Input: part model. Units: mm. Frame: model coordinates. A direction names the side the tool comes from. Coordinates: 2 decimals unless noted, no trailing zeros. Loops run counter-clockwise (first coordinate to the right, second up) from the corner with the lowest first, then second, coordinate; pieces in that order, holes last.
```python
from build123d import *

# Parameters (mm, degrees)
F0_R     = 24
F1_DEPTH = 50
F2_R     = 65
F2_R_2   = 24
F3_DEPTH = 50
F4_R     = 15


with BuildPart() as f1:
    # F0 (on Top) → F1 (new body)
    with BuildSketch(Plane.XY):
        with BuildLine():
            ThreePointArc((67.890381, 85.131845), (54.235467, 112.621108), (24.229797, 106.157675))
            ThreePointArc((24.229797, 106.157675), (0, 125), (-24.229797, 106.157675))
            ThreePointArc((-24.229797, 106.157675), (-54.235467, 112.621108), (-67.890381, 85.131845))
            ThreePointArc((-67.890381, 85.131845), (-97.728935, 77.936225), (-98.104443, 47.24461))
            ThreePointArc((-98.104443, 47.24461), (-121.865989, 27.815117), (-108.887717, 0))
            ThreePointArc((-108.887717, 0), (-121.865989, -27.815117), (-98.104443, -47.24461))
            ThreePointArc((-98.104443, -47.24461), (-97.728935, -77.936225), (-67.890381, -85.131845))
            ThreePointArc((-67.890381, -85.131845), (-54.235467, -112.621108), (-24.229797, -106.157675))
            ThreePointArc((-24.229797, -106.157675), (0, -125), (24.229797, -106.157675))
            ThreePointArc((24.229797, -106.157675), (54.235467, -112.621108), (67.890381, -85.131845))
            ThreePointArc((67.890381, -85.131845), (97.728935, -77.936225), (98.104443, -47.24461))
            ThreePointArc((98.104443, -47.24461), (121.865989, -27.815117), (108.887717, 0))
            ThreePointArc((108.887717, 0), (121.865989, 27.815117), (98.104443, 47.24461))
            ThreePointArc((98.104443, 47.24461), (97.728935, 77.936225), (67.890381, 85.131845))
        make_face()
        Circle(F0_R, mode=Mode.SUBTRACT)
    extrude(amount=F1_DEPTH)

    # F2 (on face) → F3 (join)
    with BuildSketch(Plane.XY.offset(50)):
        Circle(F2_R)
        Circle(F2_R_2, mode=Mode.SUBTRACT)
    extrude(amount=F3_DEPTH)

    # F4
    f4_edges = [f1.edges().sort_by_distance(p)[0] for p in [
        (-65, 0, 50),
        (-65, 0, 100),
    ]]
    fillet(f4_edges, radius=F4_R)


solid = f1.part
```
Item 1: Contact query for flat-ended pins moving along their axis: P1, Ø6, axis at x = 19.5, y = 38, coming from the -Z side; P2, Ø3, axis at x = -28, z = 27, coming from the -Y side; P3, Ø6, axis at y = 45.5, z = 43, coming from the +X side; P4, Ø8, axis at x = -50.5, z = 66.5, coming from the +Y side. Output: stop coordinate, or through.
Result:
P1: stops at z = 0
P2: stops at y = -110.88
P3: stops at x = 112.16
P4: stops at y = 45.42
Item 2: Line query: L1, parallel to Y at x = 0, z = 26; L2, parallel to Y at x = 0, z = 74; L3, parallel to Z at x = -101, y = 40. Output: solid intervals per line, ascending.
Result:
L1: y = -125 to -24, 24 to 125
L2: y = -65 to -24, 24 to 65
L3: z = 0 to 50
Item 3: Section query D-D (z = 7.5). Output: boundary loops of the cut face in (x, y).
Result:
outline: (-108.89, 0) arc R25 ccw to (-98.1, -47.24) arc R25 ccw to (-67.89, -85.13) arc R25 ccw to (-24.23, -106.16) arc R25 ccw to (24.23, -106.16) arc R25 ccw to (67.89, -85.13) arc R25 ccw to (98.1, -47.24) arc R25 ccw to (108.89, 0) arc R25 ccw to (98.1, 47.24) arc R25 ccw to (67.89, 85.13) arc R25 ccw to (24.23, 106.16) arc R25 ccw to (-24.23, 106.16) arc R25 ccw to (-67.89, 85.13) arc R25 ccw to (-98.1, 47.24) arc R25 ccw to start; hole circle Ø48 at (0, 0)
Item 4: Section query A-A (x = 0). Output: boundary loops of the cut face in (y, z), then the cut area to 3 significant figures.
Result:
outline: (-125, 0) - (-24, 0) - (-24, 100) - (-50, 100) arc R15 ccw to (-65, 85) - (-65, 65) arc R15 cw to (-80, 50) - (-125, 50) - close; (24, 0) - (125, 0) - (125, 50) - (80, 50) arc R15 cw to (65, 65) - (65, 85) arc R15 ccw to (50, 100) - (24, 100) - close
area: 14,200 mm2
Item 5: Section query C-C (y = -99.5). Output: boundary loops of the cut face in (x, z), then the cut area to 3 significant figures.
Result:
outline: (-66.55, 0) - (66.55, 0) - (66.55, 50) - (-66.55, 50) - close
area: 6,660 mm2
Item 6: Reachability of faces 1 (the face through (-12, -22, 100)), 2 (the face through (-2, -82, 50)) from +Z, -Z, +X, -X, +Y, -Y: full face, straight path, thin tool, end or side. Return the list, or none.
Result:
face 1: +Z, +X, -X, +Y, -Y
face 2: +Z
Item 7: Section query B-B (z = 56). Output: boundary loops of the cut face in (x, y).
Result:
outline: circle Ø136 at (0, 0); hole circle Ø48 at (0, 0)
